```python
from build123d import *

# Parameters (mm, degrees)
F0_R     = 5.861767
F1_DEPTH = 127
F2_W     = 25.4
F2_H     = 25.4
F3_DEPTH = 25.4
F4_W     = 25.4
F4_H     = 25.4
F5_DEPTH = 25.4
F7_D     = 6.35


with BuildPart() as f1:
    # F0 (on Front) → F1 (new body)
    with BuildSketch(Plane.XZ):
        with BuildLine():
            Line((-13.975801, 23.479906), (-13.975801, -40.838215))
            Line((-13.975801, -40.838215), (11.424199, -40.838215))
            Line((11.424199, -40.838215), (11.424199, 29.419485))
            Line((11.424199, 29.419485), (11.424199, 30.323507))
            ThreePointArc((11.424199, 30.323507), (10.135022, 37.425094), (6.681635, 43.762966))
            Line((6.681635, 43.762966), (-13.975801, 67.725592))
            ThreePointArc((-13.975801, 67.725592), (-33.241845, 71.538413), (-34.911566, 51.969814))
            Line((-34.911566, 51.969814), (-19.002141, 35.0763))
            ThreePointArc((-19.002141, 35.0763), (-18.691723, 34.755054), (-18.389663, 34.425937))
            ThreePointArc((-18.389663, 34.425937), (-15.225185, 29.339041), (-13.975801, 23.479906))
        make_face()
        with Locations((-25.315826, 61.006578)):
            Circle(F0_R, mode=Mode.SUBTRACT)
    extrude(amount=F1_DEPTH)

    # F2 (on face) → F3 (cut)
    with BuildSketch(Plane.XZ.offset(127)):
        with Locations((-1.275801, -28.138215)):
            Rectangle(F2_W, F2_H)
    extrude(amount=-F3_DEPTH, mode=Mode.SUBTRACT)

    # F4 (on face) → F5 (cut)
    with BuildSketch(Plane(origin=(0, 0, 0), x_dir=(-1, 0, 0), z_dir=(0, 1, 0))):
        with Locations((1.275801, -28.138215)):
            Rectangle(F4_W, F4_H)
    extrude(amount=-F5_DEPTH, mode=Mode.SUBTRACT)

    # F7 (through all)
    with Locations(Plane.XZ.offset(101.6)):
        with Locations((0, -28.686289)):
            Hole(F7_D / 2)


solid = f1.part
```
Read the model definition and answer for the solid it produces. Units are mm, in the model's axes. A direction names the side the tool comes from. Give positions to 0.01 mm unless a question says otherwise; leave off trailing zeros. Write each loop counter-clockwise with the first axis right and the second up, starting at its lowest first coordinate (ties: lowest second). Pieces come first, ordered by that corner, then holes. Notation, with made-up numbers: (84.25, -1.5) - (130.25, -1.5) arc R20 ccw to (130.25, 23.5) - close; hole circle Ø11 at (45.5, 69.5). An arc over 180 degrees is marked (long way). Write item = value, one per line. Start each with the question number.
Item 1: Find section A-A (x = 0). Give the vertices of the cut face in (y, z).
Item 2: The mould has two halves that part along X. Classify faces 1 (the flat face through (-1, -63, -40.838)), 2 (the cylindrical face through (-26.08, -62.61, 66.82)), 3 (the flat face through (-27.068, -62.611, 43.641)): +X half, -X half, draft (parallel to the pull), parting line (faces both ways), or undercut.
Item 3: Find section C-C (y = -31). State how many separate pieces and enclosed holes the cut face has, then the cut area to 3 significant figures.
Item 4: A tool of negligible diameter and unlimited length cuts with its end or side. For faces 4 (the flat face through (-13.976, -63, -1)), 5 (the flat face through (-1, -114, -15.438)), 6 (the flat face through (-8, 0, 30)), 7 (the cylindrical face through (0.688, -62.967, -31.786)), 8 (the flat face through (-1, -13, -15.438)), from which of +Z, -Z, +X, -X, +Y, -Y can it reach the whole face along a straight path? Write none if from no direction.
Item 5: Find the intervals of material crossed by probe 1 along X at (y, z) = (-29.5, -3); probe 2 along X at (y, z) = (-100.5, -27); probe 3 along Z at (x, y) = (-25, -78.5), in increasing order. Write a range as [from, to].
Item 6: Find section B-B (y = -15). Give the vertices of the cut face in (x, z), then the cut area to 3 significant figures.
Item 7: Each of these flat-tipped pins is pushed along its axis until it touches: P1, Ø8, axis at x = -5, z = -20.5, coming from the +Y side; P2, Ø10, axis at y = -64.5, z = 40.5, coming from the -X side; P3, Ø10, axis at x = -16.5, y = -71, coming from the +Z side. Where does it stop, or does it pass through?
Item 8: Find section D-D (z = 17.5). Give the vertices of the cut face in (x, y).
Response:
q1.outline = (-127, -15.44) - (-101.6, -15.44) - (-101.6, -25.51) - (-25.4, -25.51) - (-25.4, -15.44) - (0, -15.44) - (0, 51.51) - (-127, 51.51) - close; (-101.6, -40.84) - (-25.4, -40.84) - (-25.4, -31.86) - (-101.6, -31.86) - close
q2.face_1 = draft
q2.face_2 = undercut
q2.face_3 = -X half
q3.separate_pieces = 1
q3.enclosed_holes = 2
q3.area = 2,950 mm²
q4.face_4 = -Z, -X, +Y, -Y
q4.face_5 = -Z, +X, -X, -Y
q4.face_6 = +Z, -Z, +X, -X, +Y
q4.face_7 = +Y, -Y
q4.face_8 = -Z, +X, -X, +Y
q5.probe_1 = [-13.98, 11.42]
q5.probe_2 = [-13.98, -2.69], [2.69, 11.42]
q5.probe_3 = [41.45, 55.15], [66.86, 74.18]
q6.outline = (-34.91, 51.97) - (-19, 35.08) arc R17.38 cw to (-18.39, 34.43) arc R17.38 cw to (-13.98, 23.48) - (-13.98, -15.44) - (11.42, -15.44) - (11.42, 30.32) arc R22.7 ccw to (6.68, 43.76) - (-13.98, 67.73) arc R13.18 ccw (long way) to start; hole circle Ø11.72 at (-25.32, 61.01)
q6.area = 2,340 mm²
q7.P1 = -25.4
q7.P2 = -28.82
q7.P3 = 73.62
q8.outline = (-13.98, -127) - (11.42, -127) - (11.42, 0) - (-13.98, 0) - close
